Design review of the part built by this model. Coordinates are the model's own, in mm. Give positions to 0.01 mm unless a question says otherwise; leave off trailing zeros. Loops run counter-clockwise (first coordinate to the right, second up) from the corner with the lowest first, then second, coordinate; pieces in that order, holes last. Notation, with made-up numbers: (50, 89.5) -> (92, 89.5) arc R29 ccw to (92, 117.5) -> close; hole circle Ø1 at (56.5, 75). An arc over 180 degrees is marked (long way). Use a Markdown table: item, result. Add a question column.
1. For pin 1 Ø2.5 at (x, y) = (-24, 5.5) entering from -Z; pin 2 Ø1 at (x, y) = (9, 7) entering from +Z; pin 3 Ø1.5 at (y, z) = (2.5, 23) entering from -X, all flat-tipped, find the tip position at first contact; note any pin that passes through.
2. Add section A-A (x = -13). State the section outline as (y, z) points.
3. Add section C-C (y = 3.75). Count the separate pieces of the cut face and the enclosed holes in it, and give its area (3 significant figures).
4. Add section B-B (z = 10.5). State the section outline as (x, y) points, and give its area (3 significant figures).
5. To check wall thickness, follow line 1 (X direction, y = 4.25, z = 0); line 2 (X direction, y = 6.5, z = -17.5); line 3 (X direction, y = 7, z = 18.5). State the ranges of each line that lie inside material, in increasing order.
```python
from build123d import *

# Parameters (mm, degrees)
SKETCH_1_R               = 30
SKETCH_1_R_2             = 6
EXTRUDE_1_DEPTH          = 8
CUT_EXTRUDE_1_DEPTH      = 61
PATTERN_CIRCULAR_1_COUNT = 12


with BuildPart() as part:
    # Sketch 1 → Extrude 1 (new body)
    with BuildSketch(Plane(origin=(0, 0, 0), x_dir=(1, 0, 0), z_dir=(0, 1, 0))):
        with Locations(Location((0, 0, 0), (0, 0, 270))):
            Circle(SKETCH_1_R)
        with Locations(Location((0, 0, 0), (0, 0, 270))):
            Circle(SKETCH_1_R_2, mode=Mode.SUBTRACT)
    extrude(amount=EXTRUDE_1_DEPTH)

    # Sketch 2 → Cut-Extrude 1 (cut, symmetric)
    with BuildSketch(Plane(origin=(0, 0, 0), x_dir=(1, 0, 0), z_dir=(0, 1, 0))):
        with BuildLine():
            Line((21, 2), (26, 2))
            ThreePointArc((26, 2), (28, 0), (26, -2))
            Line((26, -2), (21, -2))
            ThreePointArc((21, -2), (19, 0), (21, 2))
        make_face()
    cut_extrude_1 = extrude(amount=CUT_EXTRUDE_1_DEPTH, both=True, mode=Mode.SUBTRACT)

    # Pattern Circular 1: Cut-Extrude 1 ×12 about axis
    pattern_circular_1_axis = Axis((0, 0, 0), (0, 1, 0))
    for i in range(1, PATTERN_CIRCULAR_1_COUNT):
        add(cut_extrude_1.rotate(pattern_circular_1_axis, i * 360 / PATTERN_CIRCULAR_1_COUNT), mode=Mode.SUBTRACT)


solid = part.part
```
Taken from the geometry:
| question | item | result |
|---|---|---|
| 1 | pin 1 | stops at z = -19.56 |
| 1 | pin 2 | stops at z = 28.77 |
| 1 | pin 3 | stops at x = -20.12 |
| 2 | outline | (0, -27.04) -> (8, -27.04) -> (8, -24.52) -> (0, -24.52) -> close; (0, -18.52) -> (8, -18.52) -> (8, 18.52) -> (0, 18.52) -> close; (0, 24.52) -> (8, 24.52) -> (8, 27.04) -> (0, 27.04) -> close |
| 3 | separate pieces | 1 |
| 3 | enclosed holes | 13 |
| 3 | area | 2,320 mm^2 |
| 4 | outline | (-28.1, 0) -> (-22.19, 0) -> (-22.19, 8) -> (-28.1, 8) -> close; (-16.19, 0) -> (16.19, 0) -> (16.19, 8) -> (-16.19, 8) -> close; (22.19, 0) -> (28.1, 0) -> (28.1, 8) -> (22.19, 8) -> close |
| 4 | area | 354 mm^2 |
| 5 | line 1 | x = -30 to -28, -19 to -6, 6 to 19, 28 to 30 |
| 5 | line 2 | x = -24.37 to -12.41, -8.62 to 8.62, 12.41 to 24.37 |
| 5 | line 3 | x = -23.62 to -12.99, -8.52 to 8.52, 12.99 to 23.62 |
